Geometry: see drawing. Coordinates: mm, zero at the bounding-box minimum. Round coordinates to 2 decimals unless told otherwise and drop trailing zeros. Order: outer loops, then holes, each group sorted by start corner. A loop starts at its lowest first (then second) coordinate and runs counter-clockwise, first axis right, second up. Notation, with made-up numbers: (-34.5, 21) -> (19.5, 21) arc R22 ccw to (19.5, 56) -> close; hole circle Ø8 at (45.25, 14.5). An arc over 180 degrees is marked (long way). One line per item, written item: value. Start each with the question number.
1) Section A-A (x = 15). Return the cut outline in (y, z), and give its area (3 significant figures).
2) Ray query, L1, parallel to Z at x = 16, y = 1.45; L2, parallel to Z at x = 17.75, y = 2.3 (1 decimal); L3, parallel to Z at x = 10.25, y = 1.3. Return the intervals inside material, ascending.
3) Section C-C (z = 24). Return the cut outline in (x, y).
4) Section D-D (x = 11). Return the cut outline in (y, z).
5) Section B-B (y = 1.7). Return the cut outline in (x, z).
6) Pin query (flat end, axial travel): P1, Ø2, axis at x = 20.63, z = 21.25, coming from the +Y side; P2, Ø0.9, axis at x = 28.5, y = 2, coming from the +Z side. Return the tip coordinate at first contact, or that it passes through.
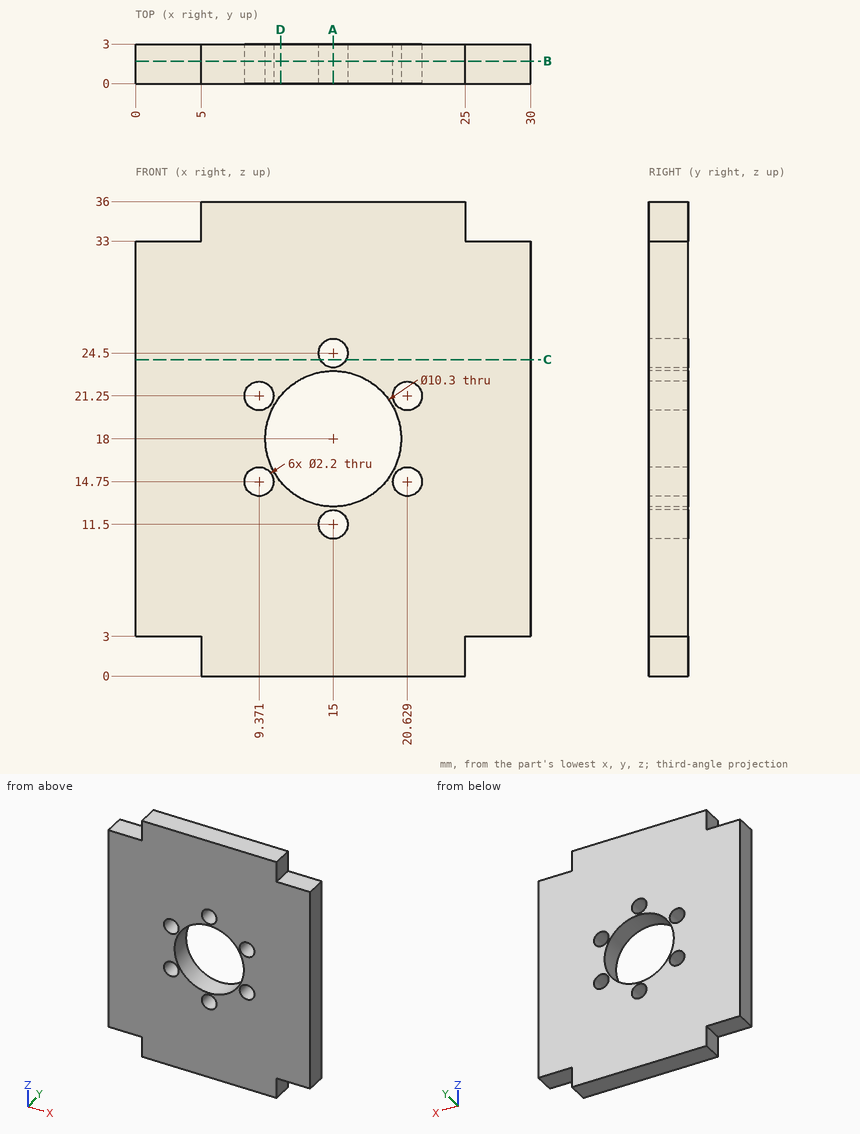
Findings:
1. outline: (0, 0) -> (3, 0) -> (3, 10.4) -> (0, 10.4) -> close; (0, 12.6) -> (3, 12.6) -> (3, 12.85) -> (0, 12.85) -> close; (0, 23.15) -> (3, 23.15) -> (3, 23.4) -> (0, 23.4) -> close; (0, 25.6) -> (3, 25.6) -> (3, 36) -> (0, 36) -> close
1. area: 63.9 mm2
2. L1: 0 to 11.04, 11.96 to 12.95, 23.05 to 24.04, 24.96 to 36
2. L2: 0 to 13.6, 22.4 to 36
2. L3: 0 to 14.09, 15.41 to 16.01, 19.99 to 20.59, 21.91 to 36
3. outline: (0, 0) -> (14.02, 0) -> (14.02, 3) -> (0, 3) -> close; (15.98, 0) -> (30, 0) -> (30, 3) -> (15.98, 3) -> close
4. outline: (0, 0) -> (3, 0) -> (3, 14.76) -> (0, 14.76) -> close; (0, 21.24) -> (3, 21.24) -> (3, 36) -> (0, 36) -> close
5. outline: (0, 3) -> (5, 3) -> (5, 0) -> (25, 0) -> (25, 3) -> (30, 3) -> (30, 33) -> (25, 33) -> (25, 36) -> (5, 36) -> (5, 33) -> (0, 33) -> close; hole circle Ø2.2 at (9.37, 14.75); hole circle Ø2.2 at (9.37, 21.25); hole circle Ø10.3 at (15, 18); hole circle Ø2.2 at (15, 11.5); hole circle Ø2.2 at (15, 24.5); hole circle Ø2.2 at (20.63, 14.75); hole circle Ø2.2 at (20.63, 21.25)
6. P1: through
6. P2: z = 33
